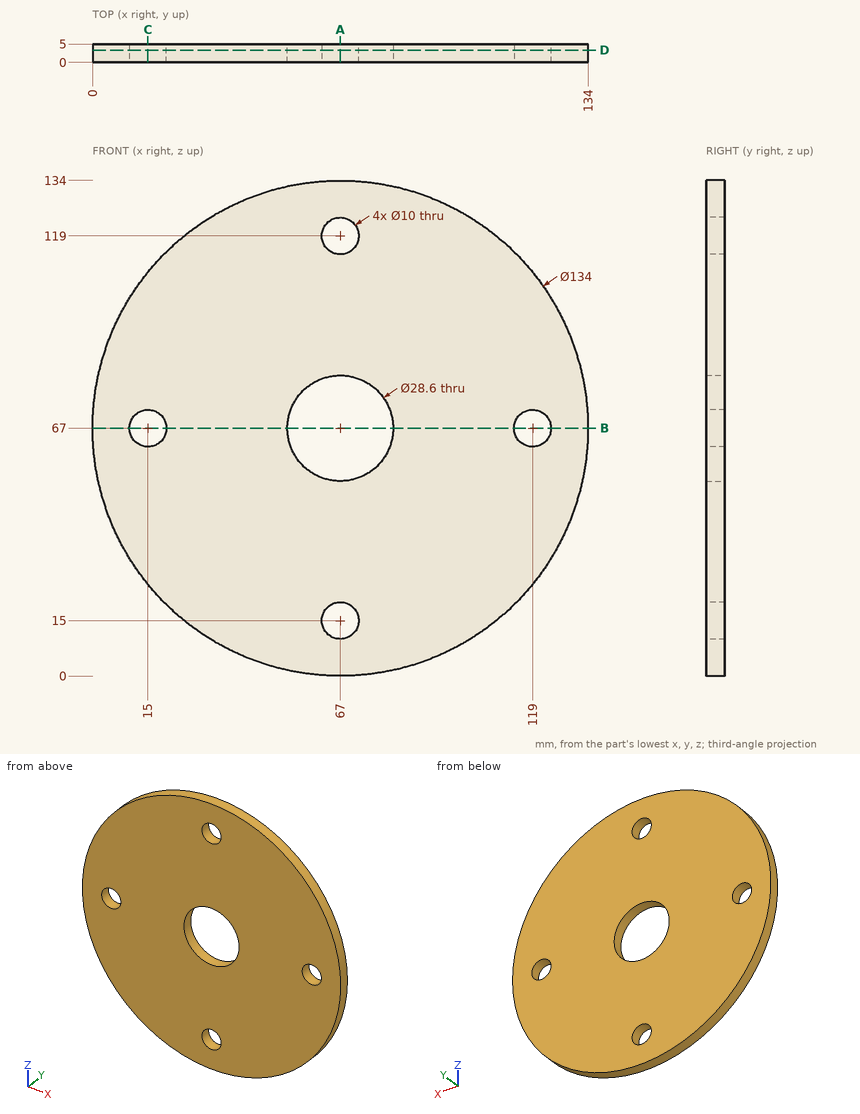
Study the drawing (mm; zero at the part's minimum x, y, z) and answer. Coordinates: 2 decimals unless noted, no trailing zeros. Loops run counter-clockwise (first coordinate to the right, second up) from the corner with the lowest first, then second, coordinate; pieces in that order, holes last. Notation, with made-up numbers: (73, 13) -> (121, 13) arc R25 ccw to (121, 49) -> close; hole circle Ø3 at (42, -2.5). An arc over 180 degrees is marked (long way). Write each question's results on one line, items separated by ' | '. Start each with the question number.
1) Flat-ended cylindrical pins translate along their axes: P1, Ø8, axis at x = 67, z = 15, coming from the -Y side; P2, Ø1, axis at y = 2.5, z = 36, coming from the -X side; P3, Ø11.5, axis at x = 119, z = 67, coming from the +Y side; P4, Ø1.5, axis at y = 3, z = 24.5, coming from the +X side. Find the tip coordinate at first contact, or state that the pin passes through.
2) Find section C-C on x = 15. Determine the outline of the cut face in (y, z), then the cut area to 3 significant figures.
3) Find section D-D on y = 3.35. Determine the outline of the cut face in (x, z).
4) Consider line 1 along Z through (x, y) = (67, 1.9); line 2 along X through (y, z) = (2.25, 121.5). Determine where each line is inside the solid, lowest interval first.
5) Find section B-B on z = 67. Determine the outline of the cut face in (x, y).
6) Find section A-A on x = 67. Determine the outline of the cut face in (y, z).
Response values:
1) P1: passes through | P2: stops at x = 7.34 | P3: stops at y = 5 | P4: stops at x = 119.4
2) outline: (0, 24.75) -> (5, 24.75) -> (5, 62) -> (0, 62) -> close; (0, 72) -> (5, 72) -> (5, 109.25) -> (0, 109.25) -> close | area: 372 mm^2
3) outline: circle Ø134 at (67, 67); hole circle Ø10 at (15, 67); hole circle Ø28.6 at (67, 67); hole circle Ø10 at (67, 15); hole circle Ø10 at (67, 119); hole circle Ø10 at (119, 67)
4) line 1: z = 0 to 10, 20 to 52.7, 81.3 to 114, 124 to 134 | line 2: x = 28.03 to 62.67, 71.33 to 105.97
5) outline: (0, 0) -> (10, 0) -> (10, 5) -> (0, 5) -> close; (20, 0) -> (52.7, 0) -> (52.7, 5) -> (20, 5) -> close; (81.3, 0) -> (114, 0) -> (114, 5) -> (81.3, 5) -> close; (124, 0) -> (134, 0) -> (134, 5) -> (124, 5) -> close
6) outline: (0, 0) -> (5, 0) -> (5, 10) -> (0, 10) -> close; (0, 20) -> (5, 20) -> (5, 52.7) -> (0, 52.7) -> close; (0, 81.3) -> (5, 81.3) -> (5, 114) -> (0, 114) -> close; (0, 124) -> (5, 124) -> (5, 134) -> (0, 134) -> close
